Input: part model. Units: mm. Frame: model coordinates. A direction names the side the tool comes from. Coordinates: 2 decimals unless noted, no trailing zeros. Answer as CSV lines item,"result". Start each with the question number.
Item 1: Draft query along Y for faces 4 (the flat face through (-36, 0, -6)), 5 (the cylindrical face through (-2.008, -42.619, -7.014)), 6 (the cylindrical face through (-18.28, -28.67, -8.74)). Return one class per face: +Y half, -Y half, draft (parallel to the pull), parting line (faces both ways), or undercut.
Item 2: First-contact query: pin 1 (1 mm diameter, centred on x = 24.5, z = -9, fed in from +Y); pin 2 (6 mm diameter, centred on x = 0, y = 40, fed in from -Z); pin 3 (9 mm diameter, centred on x = -2, y = 42, fed in from +Z); pin 4 (1 mm diameter, centred on y = -6.5, z = -2.5, fed in from -X). Flat tips, straight axial feed; report the tip coordinate or a pass-through.
Item 3: Material intervals for line 1 along Z through (x, y) = (5, -26.5); line 2 along Y through (x, z) = (-3.5, -2); line 3 along Y through (x, z) = (19, -6), sorted ascending.
Item 4: Section A-A (x = 0). State how many separate pieces and enclosed holes the cut face has, and give its area (3 significant figures).
Item 5: Access query for faces 1 (the flat face through (-7, 25, -8)), 2 (the cylindrical face through (2.008, 42.619, -7.014)), 3 (the cylindrical face through (0.242, -45.495, -3.042)). Directions: +Z, -Z, +X, -X, +Y, -Y. A direction counts if a zero-diameter tool reaches every point of the face in a straight line with its end or side. Return the directions, or none.
Autodesk Inventor part; units mm, degrees
ref_plane "YZ Plane" through (0, 0, 0) normal (1, 0, 0) x (0, 1, 0)
ref_plane "XZ Plane" through (0, 0, 0) normal (0, 1, 0) x (-1, 0, 0)
ref_plane "XY Plane" through (0, 0, 0) normal (0, 0, 1) x (1, 0, 0)
sketch "Esboço1" plane through (0, 0, 0) normal (0, 0, 1) x (1, 0, 0)
  circle A0 centre (0, 0) radius 24.5
  circle A1 centre (0, 0) radius 47.5
  dimension "d0" = 49
  dimension "d1" = 95
extrude "Extrusão1" add sketch "Esboço1" against normal blind 8
sketch "Esboço2" plane through (0, 0, -8) normal (0, 0, -1) x (-1, 0, 0)
  circle A0 centre (0, 0) radius 24.5
  circle A1 centre (0, 0) radius 30
  circle A2 centre (0, 0) radius 34
  dimension "d4" = 60
  dimension "d5" = 68
extrude "Extrusão2" add sketch "Esboço2" along normal blind 2 contours A2
sketch "Esboço3" plane through (0, 0, 0) normal (0, 0, 1) x (1, 0, 0)
  circle A0 centre (0, 0) radius 47.5
  point P0 (0, 40)
  dimension "d8" = 40
hole "Furo1" at (0, 40, 0) direction (0, 0, -1) diameter 6.6 depth 10 tip angle 118 counterbore diameter 11 counterbore depth 6
pattern_circular "Padrão circular1" count 4 over 360 about axis through (0, 0, -10) along (0, 0, 1) of "Furo1"
chamfer "Chanfro1" distance 0.5 angle 45 6 edges at (-24.5, 0, 0) (-24.5, 0, -8) (-47.5, 0, 0) (-47.5, 0, -8) (34, 0, -10) (30, 0, -10)
Determined:
1,face 4,"undercut"
1,face 5,"undercut"
1,face 6,"parting line"
2,pin 1,"stops at y = 24.08"
2,pin 2,"passes through"
2,pin 3,"stops at z = 0"
2,pin 4,"stops at x = -47.12"
3,line 1,"z = -8 to 0"
3,line 2,"y = -47.37 to -44.24, -35.76 to -24.25, 24.25 to 35.76, 44.24 to 47.37"
3,line 3,"y = -43.53 to -15.47, 15.47 to 43.53"
4,separate pieces,"4"
4,enclosed holes,"0"
4,area,"224 mm^2"
5,face 1,"-Z"
5,face 2,"+Z, -Z"
5,face 3,"+Z"
